from build123d import *

# Parameters (mm, degrees)
SKETCH_1_R          = 23
EXTRUDE_1_DEPTH     = 8
SKETCH_2_R          = 9
EXTRUDE_2_DEPTH     = 2
SKETCH_3_R          = 9
EXTRUDE_3_DEPTH     = 21
SKETCH_4_R          = 13.5
EXTRUDE_4_DEPTH     = 12
SKETCH_5_R          = 7.5
CUT_EXTRUDE_1_DEPTH = 4
SKETCH_6_R          = 5.25
CUT_EXTRUDE_2_DEPTH = 100


with BuildPart() as part:
    # Эскиз1 → Бобышка-Вытянуть1 (new body)
    with BuildSketch(Plane.XY):
        Circle(SKETCH_1_R)
    extrude(amount=EXTRUDE_1_DEPTH)

    # Эскиз2 → Бобышка-Вытянуть2 (add)
    with BuildSketch(Plane.XY.offset(8)):
        Circle(SKETCH_2_R)
    extrude(amount=EXTRUDE_2_DEPTH)

    # Эскиз3 → Бобышка-Вытянуть3 (add)
    with BuildSketch(Plane(origin=(0, 0, 0), x_dir=(-1, 0, 0), z_dir=(0, 0, -1))):
        Circle(SKETCH_3_R)
    extrude(amount=EXTRUDE_3_DEPTH)

    # Эскиз4 → Бобышка-Вытянуть4 (add)
    with BuildSketch(Plane(origin=(0, 0, -21), x_dir=(-1, 0, 0), z_dir=(0, 0, -1))):
        Circle(SKETCH_4_R)
    extrude(amount=EXTRUDE_4_DEPTH)

    # Эскиз5 → Вырез-Вытянуть1 (cut)
    with BuildSketch(Plane(origin=(0, 0, -33), x_dir=(-1, 0, 0), z_dir=(0, 0, -1))):
        Circle(SKETCH_5_R)
    extrude(amount=-CUT_EXTRUDE_1_DEPTH, mode=Mode.SUBTRACT)

    # Эскиз6 → Вырез-Вытянуть2 (cut)
    with BuildSketch(Plane(origin=(0, 0, -29), x_dir=(-1, 0, 0), z_dir=(0, 0, -1))):
        Circle(SKETCH_6_R)
    extrude(amount=-CUT_EXTRUDE_2_DEPTH, mode=Mode.SUBTRACT)


solid = part.part
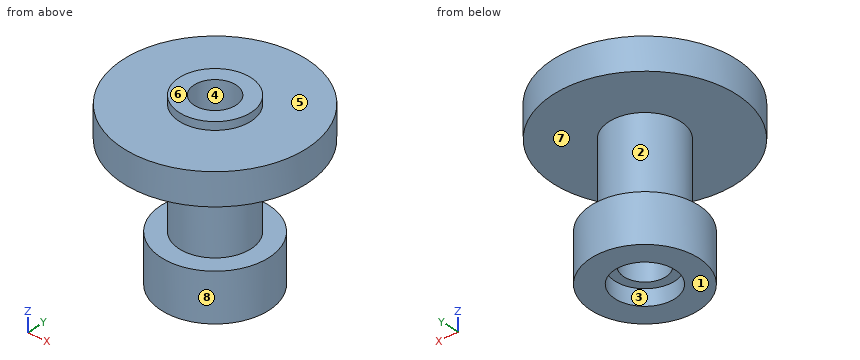
For this review, take the finished solid that the model builds, in its own axes (mm). Face numbers are marked on the shaded views. A direction names the side the tool comes from. Round coordinates to 2 decimals unless told otherwise and drop trailing zeros. Loops run counter-clockwise (first coordinate to the right, second up) from the corner with the lowest first, then second, coordinate; pieces in that order, holes last. Notation, with made-up numbers: (6.5, 85) - (64.5, 85) arc R13 cw to (64.5, 96) - close; hole circle Ø3 at (33, -40). An arc over 180 degrees is marked (long way). One line per item, written item: value. Start each with the question number.
Item 1: For L1, parallel to Z at x = 10.5, y = -3; L2, parallel to Y at x = 0, z = -30; L3, parallel to Z at x = -14, y = 3.5, list the stretches that pass through material, from the lowest coordinate up.
Item 2: Take a section at A-A (x = 0). Give the boundary of the cut face in (y, z), plus the area to 4 significant figures.
Item 3: Take a section at C-C (z = -23). Give the boundary of the cut face in (x, y).
Item 4: For the marked faces 5, 6, 7 and 8, list the 3-axis set-ups (+Z, -Z, +X, -X, +Y, -Y) from which the entire face can be reached by the end or side of a thin tool; tool diameter is ignored.
Item 5: Clearance check with flat-ended pins moving along their axes: pin 1 Ø1 at (x, z) = (-7, -6) entering from +Y; pin 2 Ø6 at (x, z) = (7, -15) entering from +Y; pin 3 Ø12 at (y, z) = (11, -8.5) entering from +X; pin 4 Ø6.5 at (x, y) = (0, 0) entering from -Z. State where each tip first meets the part, or that it passes through.
Item 6: Take a section at D-D (x = -12). Give the boundary of the cut face in (y, z), plus the area to 3 significant figures.
Item 7: The part is to be moulded in two halves that separate along Y. For the marked faces 1, 2, 3 and 4, say which applies: +Y half, -Y half, draft (parallel to the pull), parting line (faces both ways), or undercut.
Answer below:
1. L1: z = -33 to -21, 0 to 8
1. L2: y = -13.5 to -7.5, 7.5 to 13.5
1. L3: z = 0 to 8
2. outline: (-23, 0) - (-9, 0) - (-9, -21) - (-13.5, -21) - (-13.5, -33) - (-7.5, -33) - (-7.5, -29) - (-5.25, -29) - (-5.25, 10) - (-9, 10) - (-9, 8) - (-23, 8) - close; (5.25, -29) - (7.5, -29) - (7.5, -33) - (13.5, -33) - (13.5, -21) - (9, -21) - (9, 0) - (23, 0) - (23, 8) - (9, 8) - (9, 10) - (5.25, 10) - close
2. area: 636.5 mm2
3. outline: circle Ø27 at (0, 0); hole circle Ø10.5 at (0, 0)
4. face 5: +Z
4. face 6: +Z, +X, -X, +Y, -Y
4. face 7: none
4. face 8: -Z
5. pin 1: stops at y = 6.22
5. pin 2: stops at y = 8.06
5. pin 3: stops at x = 7.48
5. pin 4: passes through
6. outline: (-19.62, 0) - (19.62, 0) - (19.62, 8) - (-19.62, 8) - close; (-6.18, -33) - (6.18, -33) - (6.18, -21) - (-6.18, -21) - close
6. area: 462 mm2
7. face 1: draft
7. face 2: parting line
7. face 3: undercut
7. face 4: undercut
